Source: CAD feature listing. Evaluate the final solid. Frame: model axes, mm. A direction names the side the tool comes from. Round coordinates to 2 decimals unless told otherwise and drop trailing zeros. Loops run counter-clockwise (first coordinate to the right, second up) from the corner with the lowest first, then second, coordinate; pieces in that order, holes last. Notation, with made-up numbers: (35.5, 4.25) - (82.5, 4.25) arc R14 ccw to (82.5, 30.25) - close; hole circle Ø7 at (31.5, 38.5). An arc over 180 degrees is marked (long way). Write item = value, one per line. Start each with the question number.
from build123d import *

# Parameters (mm, degrees)
BOSS_EXTRUDE1_DEPTH     = 9
SKETCH2_R               = 6.5
CUT_EXTRUDE1_DEPTH      = 2.5
SKETCH3_R               = 4.5
CUT_EXTRUDE2_DEPTH      = 20
FILLET1_R               = 4
SKETCH4_R               = 6.5
CUT_EXTRUDE3_DEPTH      = 20
CUT_EXTRUDE3_DEPTH_BACK = 12.5
SKETCH6_R               = 2
CUT_EXTRUDE4_DEPTH      = 10


with BuildPart() as part:
    # Sketch1 → Boss-Extrude1 (new body)
    with BuildSketch(Plane(origin=(0, 0, 0), x_dir=(1, 0, 0), z_dir=(0, 1, 0))):
        Polygon((-19, 11.5), (-19, -19), (19, -19), (19, 11.5), (11.5, 11.5), (11.5, -11.5), (-11.5, -11.5), (-11.5, 11.5), align=None)
    extrude(amount=BOSS_EXTRUDE1_DEPTH)

    # Sketch2 → Cut-Extrude1 (cut, symmetric)
    with BuildSketch(Plane(origin=(15.25, 0, 0), x_dir=(0, 0, -1), z_dir=(1, 0, 0))):
        with Locations((0, 9)):
            Circle(SKETCH2_R)
    cut_extrude1 = extrude(amount=CUT_EXTRUDE1_DEPTH, both=True, mode=Mode.SUBTRACT)

    # Sketch3 → Cut-Extrude2 (cut, through all)
    with BuildSketch(Plane(origin=(0, 0, 0), x_dir=(0, 0, -1), z_dir=(1, 0, 0))):
        with Locations((0, 9)):
            Circle(SKETCH3_R)
    cut_extrude2 = extrude(amount=CUT_EXTRUDE2_DEPTH, mode=Mode.SUBTRACT)

    # Mirror1: Cut-Extrude1, Cut-Extrude2 across plane
    add(cut_extrude1.mirror(Plane(origin=(0, 0, 0), x_dir=(0, 0, 1), z_dir=(1, 0, 0))), mode=Mode.SUBTRACT)
    add(cut_extrude2.mirror(Plane(origin=(0, 0, 0), x_dir=(0, 0, 1), z_dir=(1, 0, 0))), mode=Mode.SUBTRACT)

    # Fillet1
    fillet1_edges = [part.edges().sort_by_distance(p)[0] for p in [
        (19, 0, 3.75),
        (-19, 0, 3.75),
    ]]
    fillet(fillet1_edges, radius=FILLET1_R)

    # Sketch4 → Cut-Extrude3 (cut, two sides)
    with BuildSketch(Plane.XY) as cut_extrude3_sk:
        with Locations((0, 9)):
            Circle(SKETCH4_R)
    extrude(amount=CUT_EXTRUDE3_DEPTH, mode=Mode.SUBTRACT)
    extrude(cut_extrude3_sk.sketch, amount=-CUT_EXTRUDE3_DEPTH_BACK, mode=Mode.SUBTRACT)

    # Sketch6 → Cut-Extrude4 (cut, through all)
    with BuildSketch(Plane(origin=(0, 9, 0), x_dir=(1, 0, 0), z_dir=(0, 1, 0))):
        with Locations((-15.5, 9)):
            Circle(SKETCH6_R)
        with Locations((15.5, 9)):
            Circle(SKETCH6_R)
        with Locations((15.5, -15.5)):
            Circle(SKETCH6_R)
        with Locations((-15.5, -15.5)):
            Circle(SKETCH6_R)
    extrude(amount=-CUT_EXTRUDE4_DEPTH, mode=Mode.SUBTRACT)


solid = part.part
(1) Access query for faces 4 (the face through (11.5, 4, 0)), 5 (the face through (15.3, 2.5, 0.1)), 6 (the face through (-15, 4, -11.5)). Directions: +Z, -Z, +X, -X, +Y, -Y. A direction counts if a zero-diameter tool reaches every point of the face in a straight line with its end or side. Return the directions, or none.
(2) Material intervals for line 1 along Z through (x, y) = (15.5, 2.25); line 2 along X through (y, z) = (7.25, -9); line 3 along Z through (x, y) = (-15.5, 7), sorted ascending. Write a range as from..to.
(3) Cut plane B-B (y = 3.5). Output: boundary loops of the cut face in (x, z), and give its area (3 significant figures).
(4) Mould query, pull axis X, two halves, no side actions, for faces 1 (the face through (17.797, 1.141, 3.536)), 2 (the face through (14, 9, -7)), 3 (the face through (-15.3, 2.5, 0.1)). Classes: +X half, -X half, draft (parallel to the pull), parting line (faces both ways), or undercut.
(5) Cut plane A-A (z = 0). Output: boundary loops of the cut face in (x, y), and give its area (3 significant figures).
(6) Cut plane D-D (x = 15.5). Output: boundary loops of the cut face in (y, z), and give its area (3 significant figures).
(7) Cut plane C-C (z = 15). Output: boundary loops of the cut face in (x, y).
(8) Pin query (flat end, axial travel): P1, Ø1.5, axis at y = 1.5, z = 7, coming from the +X side; P2, Ø6.5, axis at x = 15.5, z = 15.5, coming from the -Y side. Return the tip coordinate at first contact, or that it passes through.
Solution:
q1.face_4 = -Z, +Y, -Y
q1.face_5 = +Y
q1.face_6 = -Z, +X, -X, +Y, -Y
q2.line_1 = -11.5..-11, -7..13.5, 17.5..19
q2.line_2 = -19..-17.5, -13.5..-11.5, 11.5..13.5, 17.5..19
q2.line_3 = -11.5..-11, -7..-6.18, 6.18..13.5, 17.5..19
q3.outline = (-18.97, -11.5) - (-11.5, -11.5) - (-11.5, 11.5) - (-3.46, 11.5) - (-3.46, 19) - (-18.97, 19) - close; (3.46, 11.5) - (11.5, 11.5) - (11.5, -11.5) - (18.97, -11.5) - (18.97, 19) - (3.46, 19) - close; hole (-17.75, -3.46) - (-12.75, -3.46) - (-12.75, 3.46) - (-17.75, 3.46) - close; hole circle Ø4 at (-15.5, -9); hole circle Ø4 at (-15.5, 15.5); hole (12.75, -3.46) - (17.75, -3.46) - (17.75, 3.46) - (12.75, 3.46) - close; hole circle Ø4 at (15.5, -9); hole circle Ø4 at (15.5, 15.5)
q3.area = 457 mm^2
q4.face_1 = +X half
q4.face_2 = draft
q4.face_3 = undercut
q5.outline = (-19, 4) arc R4 ccw to (-15, 0) - (-11.5, 0) - (-11.5, 4.5) - (-12.75, 4.5) - (-12.75, 2.5) - (-17.75, 2.5) - (-17.75, 4.5) - (-19, 4.5) - close; (11.5, 0) - (15, 0) arc R4 ccw to (19, 4) - (19, 4.5) - (17.75, 4.5) - (17.75, 2.5) - (12.75, 2.5) - (12.75, 4.5) - (11.5, 4.5) - close
q5.area = 40.6 mm^2
q6.outline = (0.03, -11.5) - (9, -11.5) - (9, -11) - (0.03, -11) - close; (0.03, -7) - (9, -7) - (9, -6.5) arc R6.5 cw to (9, 6.5) - (9, 13.5) - (0.03, 13.5) - close; (0.03, 17.5) - (9, 17.5) - (9, 19) - (0.03, 19) - close
q6.area = 135 mm^2
q7.outline = (-19, 4) arc R4 ccw to (-17.44, 0.83) - (-17.44, 9) - (-19, 9) - close; (-13.56, 0) - (13.56, 0) - (13.56, 9) - (6.5, 9) arc R6.5 cw to (-6.5, 9) - (-13.56, 9) - close; (17.44, 0.83) arc R4 ccw to (19, 4) - (19, 9) - (17.44, 9) - close
q8.P1 = 18.6
q8.P2 = 0
